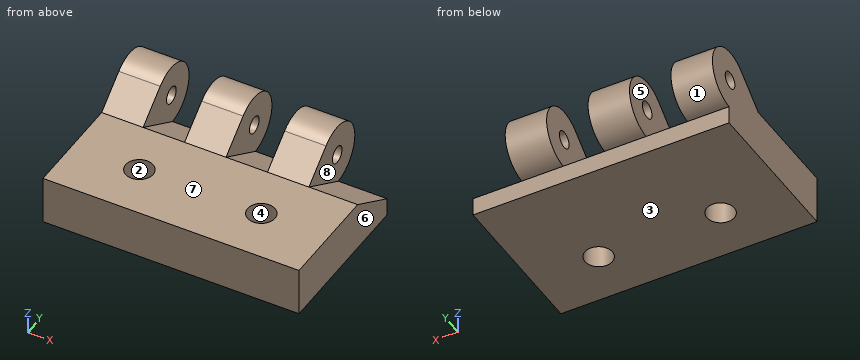
Autodesk Fusion 360 part; units mm, degrees
sketch "Sketch1" plane through (0, 0, 0) normal (0, 0, 1) x (1, 0, 0)
  line L0 (21, 8.5) -> (-21, 8.5)
  line L1 (-21, 8.5) -> (-21, -8.5)
  line L2 (-21, -8.5) -> (21, -8.5)
  line L3 (21, -8.5) -> (21, 8.5)
  line L4 (21, 8.5) -> (-21, -8.5) construction
  line L5 (-21, 8.5) -> (21, -8.5) construction
  dimension "d1" = 17
  dimension "d2" = 42
extrude "Extrude1" add sketch "Sketch1" along normal blind 8
sketch "Sketch2" plane through (0, 0, 8) normal (0, 0, 1) x (-1, 0, 0)
  line L0 (-21, 8.5) -> (-21, -8.5)
  line L1 (-21, -8.5) -> (21, -8.5)
  line L2 (21, -8.5) -> (21, 8.5)
  line L3 (21, 8.5) -> (-21, 8.5)
  circle A0 centre (14, 0) radius 3.15
  circle A1 centre (-14, 0) radius 3.15
  dimension "d6" = 6.3
  dimension "d7" = 6.3
  dimension "d8" = 28
  dimension "d9" = 7
sketch "Sketch3" plane through (21, 0, 0) normal (1, 0, 0) x (0, 1, 0)
  line L0 (-8.5, 0) -> (8.5, 0)
  line L1 (8.5, 0) -> (8.5, 8)
  line L2 (8.5, 8) -> (-8.5, 8)
  line L3 (-8.5, 8) -> (-8.5, 0)
  line L4 (8.5, 8) -> (17, 3)
  line L5 (17, 3) -> (17, 0)
  line L6 (17, 0) -> (8.5, 0)
  dimension "d23" = 8.5
  dimension "d24" = 3
extrude "Extrude3" add sketch "Sketch3" against normal up to surface (42 mm away) contours L1 L4 L5 L6
sketch "Sketch4" plane through (-21, 0, 0) normal (-1, 0, 0) x (0, -1, 0)
  line L0 (-17, 0) -> (8.5, 0)
  line L1 (8.5, 0) -> (8.5, 8)
  line L2 (8.5, 8) -> (-8.5, 8)
  line L3 (-8.5, 8) -> (-17, 3)
  line L4 (-17, 3) -> (-17, 0)
  line L5 (-8.5, 8) -> (-13.4696, 12.057)
  arc A0 (-13.4696, 12.057) -> (-17, 3) centre (-16.7002, 8.0997) ccw
extrude "Extrude4" add sketch "Sketch4" against normal blind 6.8 contours L3 L5 A0
extrude "Extrude5" add 1 faces at (-14.2, 12.9899, 7.6857) along direction (1, 0, 0) blind 6.8 from surface at 6.8
extrude "Extrude6" add 1 faces at (-0.6, 12.9899, 7.6857) along direction (1, 0, 0) blind 6.8 from surface at 6.8
sketch "Sketch5" plane through (-21, 0, 0) normal (-1, 0, 0) x (0, -1, 0)
  line L0 (-17, 0) -> (8.5, 0)
  line L1 (8.5, 0) -> (8.5, 8)
  line L2 (8.5, 8) -> (-8.5, 8)
  line L3 (-8.5, 8) -> (-13.4696, 12.057)
  arc A0 (-13.4696, 12.057) -> (-17, 3) centre (-16.7002, 8.0997) ccw
  line L4 (-17, 3) -> (-17, 0)
  circle A1 centre (-16.7002, 8.0997) radius 1.4
  dimension "d35" = 2.8
extrude "Extrude7" cut sketch "Sketch5" against normal up to surface (34 mm away) contours A1
sketch "Sketch8" plane through (0, 0, 8) normal (0, 0, 1) x (-1, 0, 0)
  line L0 (-21, 8.5) -> (-21, -8.5)
  line L1 (-21, -8.5) -> (-13, -8.5)
  line L2 (-13, -8.5) -> (-6.2, -8.5)
  line L3 (-6.2, -8.5) -> (0.6, -8.5)
  line L4 (0.6, -8.5) -> (7.4, -8.5)
  line L5 (7.4, -8.5) -> (14.2, -8.5)
  line L6 (14.2, -8.5) -> (21, -8.5)
  line L7 (21, -8.5) -> (21, 8.5)
  line L8 (21, 8.5) -> (-21, 8.5)
  line L9 (21, 0) -> (-21, 0) construction
  circle A0 centre (10, 0) radius 2.25 construction
  circle A1 centre (-10, 0) radius 2.25 construction
  dimension "d49" = 20
  dimension "d50" = 4.5
  dimension "d51" = 11
  dimension "d52" = 11
hole "Hole3" at (-10, 0, 8) at (10, 0, 8) direction (0, 0, -1) diameter 4.5 depth 10 tip angle 118
Verification items for the finished model (mm, model axes). Face numbers are marked on the shaded views. A direction names the side the tool comes from. Coordinates: 2 decimals unless noted, no trailing zeros. Order: outer loops, then holes, each group sorted by start corner. A loop starts at its lowest first (then second) coordinate and runs counter-clockwise, first axis right, second up. Notation, with made-up numbers: (52, 56) -> (101, 56) arc R18 ccw to (101, 86) -> close; hole circle Ø11 at (25, -11). An arc over 180 degrees is marked (long way). Put each result on its own line as item: value. Start each with the question number.
1) Cross-section at A-A (y = 0). Enter the section's corners in (x, z), plus the area to 3 significant figures.
2) Tool access check on the marked faces 5, 6, 7 and 8. Record the directions out of +Z, -Z, +X, -X, +Y, -Y that give a thin tool (end or side, any length) a straight path to the whole face; none if there is none.
3) Release check for a two-part mould opening along Y. For the marked faces 1, 2, 3 and 4 record: pulls with the +Y half, pulls with the -Y half, needs draft (parallel to the pull), parting line crosses it, or undercut.
4) Cross-section at B-B (x = -10). Enter the section's corners in (y, z), plus the area to 3 significant figures.
5) Go/stop test with flat-tipped pins: pin 1 (5 mm diameter, centred on y = 17, z = 10.5, fed in from +X); pin 2 (6 mm diameter, centred on x = -14, z = 2, fed in from +Y). Record where each tip stops, or that it passes through.
6) Cross-section at C-C (x = 10). Enter the section's corners in (y, z).
7) Cross-section at D-D (y = 16). Enter the section's corners in (x, z), plus the area to 3 significant figures.
8) Material ranges on L1, parallel to X at y = 13, z = 7.5; L2, parallel to X at y = 0, z = 2.5; L3, parallel to Z at x = 17, y = 6, recorded low to high.
Geometry check:
1. outline: (-21, 0) -> (-12.25, 0) -> (-12.25, 8) -> (-21, 8) -> close; (-7.75, 0) -> (7.75, 0) -> (7.75, 8) -> (-7.75, 8) -> close; (12.25, 0) -> (21, 0) -> (21, 8) -> (12.25, 8) -> close
1. area: 264 mm^2
2. face 5: +Z, +Y
2. face 6: +Z, -Z, +X, +Y, -Y
2. face 7: +Z, +X, -X, -Y
2. face 8: +Z, +X, +Y
3. face 1: parting line crosses it
3. face 2: undercut
3. face 3: needs draft
3. face 4: undercut
4. outline: (-8.5, 0) -> (-2.25, 0) -> (-2.25, 8) -> (-8.5, 8) -> close; (2.25, 0) -> (17, 0) -> (17, 3) -> (8.5, 8) -> (2.25, 8) -> close
4. area: 147 mm^2
5. pin 1: stops at x = 13
5. pin 2: stops at y = 20.76
6. outline: (-8.5, 0) -> (-2.25, 0) -> (-2.25, 8) -> (-8.5, 8) -> close; (2.25, 0) -> (17, 0) -> (17, 3) arc R5.11 ccw (long way) to (13.47, 12.06) -> (8.5, 8) -> (2.25, 8) -> close; hole circle Ø2.8 at (16.7, 8.1)
7. outline: (-21, 0) -> (21, 0) -> (21, 3.59) -> (13, 3.59) -> (13, 6.89) -> (6.2, 6.89) -> (6.2, 3.59) -> (-0.6, 3.59) -> (-0.6, 6.89) -> (-7.4, 6.89) -> (-7.4, 3.59) -> (-14.2, 3.59) -> (-14.2, 6.89) -> (-21, 6.89) -> close; (-21, 9.31) -> (-14.2, 9.31) -> (-14.2, 13.16) -> (-21, 13.16) -> close; (-7.4, 9.31) -> (-0.6, 9.31) -> (-0.6, 13.16) -> (-7.4, 13.16) -> close; (6.2, 9.31) -> (13, 9.31) -> (13, 13.16) -> (6.2, 13.16) -> close
7. area: 297 mm^2
8. L1: x = -21 to -14.2, -7.4 to -0.6, 6.2 to 13
8. L2: x = -21 to -12.25, -7.75 to 7.75, 12.25 to 21
8. L3: z = 0 to 8
